Answer from the drawing. Dimensions are ordinates in mm from the lowest x, y and z of the part. Coordinates: 2 decimals unless noted, no trailing zeros. Order: outer loops, then holes, each group sorted by start corner. A loop starts at its lowest first (then second) coordinate and runs counter-clockwise, first axis right, second up. Notation, with made-up numbers: (-25.75, -37.75) - (-13.75, -37.75) arc R32 ccw to (-13.75, -10.75) - close; hole circle Ø7 at (-25, 6.25). An arc over 180 degrees is marked (long way). Answer as a JSON object with one key per item and string values. Group by question number.
1) Find the intervals of material crossed by line 1 along X through (y, z) = (3.15, 14.5); line 2 along Z through (x, y) = (1, 2.2); line 3 along Y through (x, z) = (4.7, 24), in increasing order.
2) This flat-tipped pin is pushed along its axis until it touches: P1, Ø2, axis at x = 1, z = 16.5, coming from the -Y side. Where does it stop, or does it pass through?
3) Section A-A (z = 39) is taken. Give the vertices of the cut face in (x, y), plus the area to 3 significant figures.
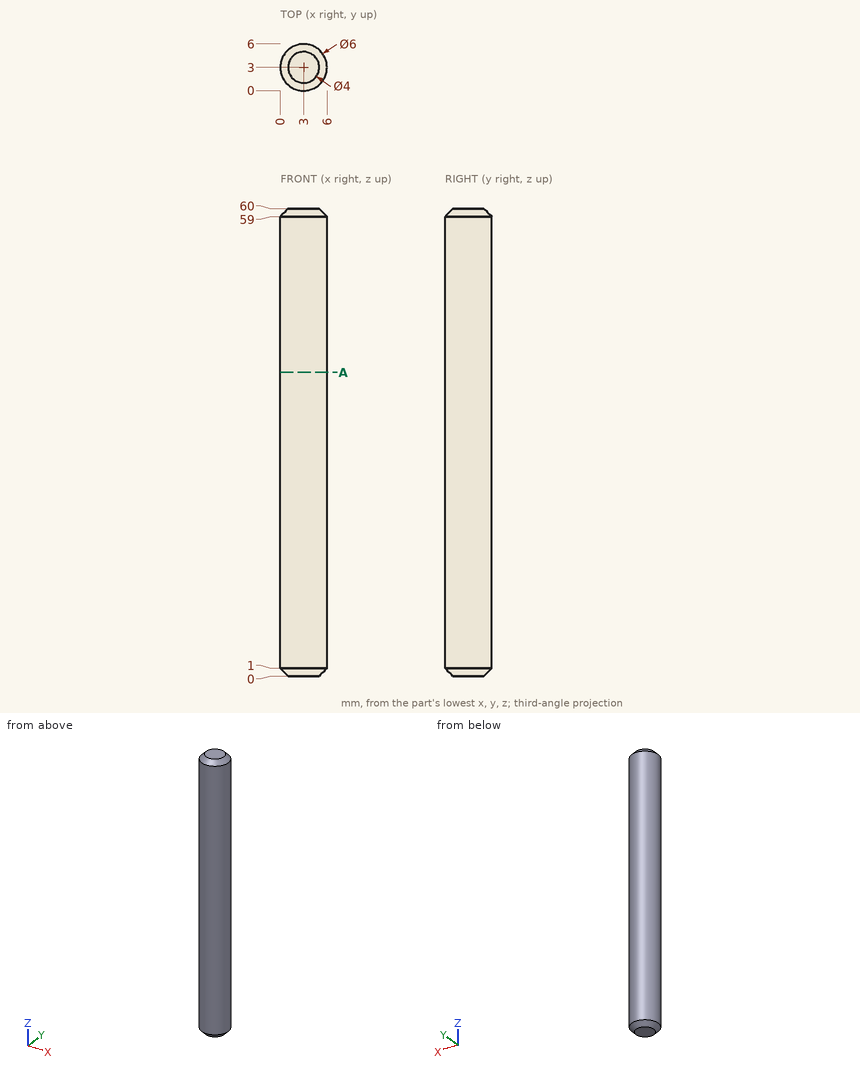
Report:
{
 "1": {"line 1": "x = 0 to 6", "line 2": "z = 0.15 to 59.85", "line 3": "y = 0.53 to 5.47"},
 "2": {"P1": "stops at y = 0.17"},
 "3": {"outline": "circle Ø6 at (3, 3)", "area": "28.3 mm²"}
}
